from build123d import *


with BuildPart() as f1:
    # F0 (on Front) → F1 (revolve)
    with BuildSketch(Plane.XZ):
        Polygon((-15.24, 0), (0, 0), (0, 25.4), (-10.009022, 25.4), align=None)
    revolve(axis=Axis((0, 0, 12.7), (0, 0, -1)))

    # F2 (on Front) → F3 (revolve)
    with BuildSketch(Plane.XZ):
        Polygon((-15.24, 76.2), (-10.009022, 25.4), (0, 25.4), (0, 76.2), align=None)
    revolve(axis=Axis((0, 0, 50.8), (0, 0, 1)))

    # F4 (on Front) → F5 (revolve)
    with BuildSketch(Plane.XZ):
        Polygon((-15.24, 76.2), (0, 76.2), (0, 88.9), align=None)
    revolve(axis=Axis((0, 0, 82.55), (0, 0, 1)))


solid = f1.part
CAD build for the part. Positions are in the model's coordinates, mm. Round coordinates to 2 decimals unless told otherwise and drop trailing zeros. Loops run counter-clockwise (first coordinate to the right, second up) from the corner with the lowest first, then second, coordinate; pieces in that order, holes last. Notation, with made-up numbers: (10.25, 8.25) - (56.25, 8.25) arc R19 ccw to (56.25, 28.25) - close; hole circle Ø11 at (69, -27). An arc over 180 degrees is marked (long way). Put each result on its own line as item: value.
1. Slice it at B-B on z = 20. List the corners of the cut face in (x, y).
Geometry check:
outline: circle Ø22.24 at (0, 0)
2. Two-plate mould, pull along Z, no slides. Class faces 1 (the flat face through (0, 0, 0)), 2 (the conical face through (2.619, -11.793, 15.344)), 3 (the conical face through (2.1, 1.6, 86.7)): released by +Z, released by -Z, zero draft, split by the parting line, or undercut.
Geometry check:
face 1: released by -Z
face 2: undercut
face 3: released by +Z
3. Pin check, flat tips, straight feed: P1, Ø6, axis at y = 2.5, z = 33.5, coming from the -X side; P2, Ø2, axis at x = 6, y = -5.5, coming from the -Z side; P3, Ø2, axis at x = 1, y = 4, coming from the +Z side; P4, Ø1.5, axis at x = -1, y = 10, coming from the +Z side. Stop position of each tip, or through.
Geometry check:
P1: x = -11.07
P2: z = 0
P3: z = 86.3
P4: z = 81.15
4. Wall check: line 1 (X direction, y = -9, z = 70.5); line 2 (Y direction, x = 7, z = 34.5); line 3 (X direction, y = 9, z = 18). Give the ranges that are in metal, low to high.
Geometry check:
line 1: -11.56 to 11.56
line 2: -8.42 to 8.42
line 3: -7.21 to 7.21
5. Slice it at A-A on z = 79.5. List the corners of the cut face in (x, y), and give its area (3 significant figures).
Geometry check:
outline: circle Ø22.56 at (0, 0)
area: 400 mm²
